```python
from build123d import *

# Parameters (mm, degrees)
SKETCH1_W           = 19.05
SKETCH1_H           = 19.05
SKETCH1_R           = 3.175
BOSS_EXTRUDE1_DEPTH = 0.79375
SKETCH2_W           = 19.05
SKETCH2_H           = 19.05
BOSS_EXTRUDE2_DEPTH = 1.5875


with BuildPart() as part:
    # Sketch1 → Boss-Extrude1 (new body, symmetric)
    with BuildSketch(Plane.XY):
        Rectangle(SKETCH1_W, SKETCH1_H)
        Circle(SKETCH1_R, mode=Mode.SUBTRACT)
    extrude(amount=BOSS_EXTRUDE1_DEPTH, both=True)

    # Sketch2 → Boss-Extrude2 (add)
    with BuildSketch(Plane.XZ.offset(9.525)):
        with Locations((0, 10.31875)):
            Rectangle(SKETCH2_W, SKETCH2_H)
    extrude(amount=-BOSS_EXTRUDE2_DEPTH)


solid = part.part
```
Work out the finished part from the listing and answer in its coordinate system (mm). A direction names the side the tool comes from. Give positions to 0.01 mm unless a question says otherwise; leave off trailing zeros. Loops run counter-clockwise (first coordinate to the right, second up) from the corner with the lowest first, then second, coordinate; pieces in that order, holes last. Notation, with made-up numbers: M -14.75,-34 L 43.25,-34 A20 cw 43.25,-16 Z; hole C 72,68.5 d2. An arc over 180 degrees is marked long. One line per item, written item: value. Start each with the question number.
1. Find section D-D (z = 12.75). Give the vertices of the cut face in (x, y) (1 decimal).
2. Find section C-C (x = -8.5). Give the vertices of the cut face in (y, z) (1 decimal).
3. Which of the six approach directions +Z, -Z, +X, -X, +Y, -Y give full straight-line access (tool end or side, diameter ignored) to faces 1 (the face through (0, -7.938, 10)), 2 (the face through (9.525, -9, 5))?
4. Find section A-A (x = 0). Give the vertices of the cut face in (y, z) (1 decimal).
5. Find the intervals of material crossed by probe 1 along Y at (x, z) = (0, 0.25) (3 decimals); probe 2 along Z at (x, y) = (-1.25, -5.5); probe 3 along Y at (x, z) = (0, 3.5) (1 decimal), in increasing order.
6. Each of these flat-tipped pins is pushed along its axis until it touches: P1, Ø7.5, axis at x = 0, y = 0, coming from the +Z side; P2, Ø9.5, axis at x = -4, z = 13, coming from the +Y side. Where does it stop, or does it pass through?
7. Find section B-B (y = 0). Give the vertices of the cut face in (x, z) (3 decimals).
Reported:
1. outline: M -9.5,-9.5 L 9.5,-9.5 L 9.5,-7.9 L -9.5,-7.9 Z
2. outline: M -9.5,-0.8 L 9.5,-0.8 L 9.5,0.8 L -7.9,0.8 L -7.9,19.8 L -9.5,19.8 Z
3. face 1: +Z, +X, -X, +Y
3. face 2: +Z, -Z, +X, +Y, -Y
4. outline: M -9.5,-0.8 L -3.2,-0.8 L -3.2,0.8 L -7.9,0.8 L -7.9,19.8 L -9.5,19.8 Z; M 3.2,-0.8 L 9.5,-0.8 L 9.5,0.8 L 3.2,0.8 Z
5. probe 1: y = -9.525 to -3.175, 3.175 to 9.525
5. probe 2: z = -0.79 to 0.79
5. probe 3: y = -9.5 to -7.9
6. P1: stops at z = 0.79
6. P2: stops at y = -7.94
7. outline: M -9.525,-0.794 L -3.175,-0.794 L -3.175,0.794 L -9.525,0.794 Z; M 3.175,-0.794 L 9.525,-0.794 L 9.525,0.794 L 3.175,0.794 Z
